Build history of the part. All positions in model axes, mm. A direction names the side the tool comes from. Round coordinates to 2 decimals unless told otherwise and drop trailing zeros. Loops run counter-clockwise (first coordinate to the right, second up) from the corner with the lowest first, then second, coordinate; pieces in that order, holes last. Notation, with made-up numbers: (21.25, 42.25) -> (40.25, 42.25) arc R14 cw to (40.25, 59.25) -> close; hole circle Ø9 at (-6.75, 19). An arc over 180 degrees is marked (long way). Put each result on its own line as item: value. Start each with the question number.
Item 1: Cut at A-A, the plane y = 0. List the corners of the cut face in (x, z), plus the area to 3 significant figures.
Item 2: Cut at C-C, the plane z = 0.75. Count the separate pieces of the cut face and the enclosed holes in it, plus the area to 3 significant figures.
Item 3: Tool access for faces 4 (the cylindrical face through (-2.664, -13.159, 1.479)), 5 (the cylindrical face through (-11.995, -5.952, 1.479)), 6 (the flat face through (8, 2, 3)), 7 (the flat face through (8.631, -0.183, 1.479)): list every direction of +Z, -Z, +X, -X, +Y, -Y with a clear straight run to the whole face (end or side of a thin tool).
Item 4: Cut at B-B, the plane x = 11. List the corners of the cut face in (y, z).
Item 5: Pull direction Y, two halves, no side cores. Call faces 1 (the cylindrical face through (-10.046, -8.853, 1.479)), 2 (the flat face through (37.972, -12.897, 1.479)), 3 (the flat face through (27.025, -3.925, 1.479)): +Y half, -Y half, draft (parallel to the pull), parting line (faces both ways), or undercut.
Item 6: Drill centre lines: probe 1 along Y at (x, z) = (20, 0.35); probe 2 along X at (y, z) = (0, 1.25); probe 3 along X at (y, z) = (2.75, 2.7). Where is each one in solid material? Low to high. Write a range as [from, to].
Item 7: Flat gauge pins, fed straight in: pin 1 Ø1 at (x, z) = (20, 2) entering from +Y; pin 2 Ø0.9 at (x, z) = (21, 1.5) entering from -Y; pin 3 Ø1 at (y, z) = (-6.5, 1.5) entering from -X; pin 4 Ø2.5 at (x, y) = (41.23, -11.45) entering from -Z. Where does each tip first touch, or does it go through?
```python
from build123d import *

# Parameters (mm, degrees)
SKETCH2_R           = 1.5
BOSS_EXTRUDE2_DEPTH = 3
CUT_EXTRUDE2_DEPTH  = 3


with BuildPart() as part:
    # Sketch2 → Boss-Extrude2 (new body)
    with BuildSketch(Plane.XY):
        with BuildLine():
            Line((33.856406461, -4.911436862), (20, -2.911436862))
            Line((20, -2.911436862), (8.072676136, 9))
            ThreePointArc((8.072676136, 9), (-5.877422545, 10.565226179), (-11.903927815, -2.112960617))
            ThreePointArc((-11.903927815, -2.112960617), (-13.14288127, -2.654199937), (-14.208555951, -3.486235477))
            ThreePointArc((-14.208555951, -3.486235477), (-14.131494839, -3.78652263), (-14.048088143, -4.085109489))
            ThreePointArc((-14.048088143, -4.085109489), (-12.709169027, -4.272836063), (-11.365584201, -4.122086336))
            ThreePointArc((-11.365584201, -4.122086336), (-11.169703548, -4.626642697), (-10.951436862, -5.12192646))
            ThreePointArc((-10.951436862, -5.12192646), (-12.008090957, -5.965388247), (-12.82210701, -7.044889767))
            ThreePointArc((-12.82210701, -7.044889767), (-12.669951657, -7.315), (-12.51210701, -7.581825517))
            ThreePointArc((-12.51210701, -7.581825517), (-11.170223244, -7.416617696), (-9.911436862, -6.9232593))
            ThreePointArc((-9.911436862, -6.9232593), (-9.591641884, -7.359925677), (-9.252623584, -7.781841479))
            ThreePointArc((-9.252623584, -7.781841479), (-10.05496909, -8.870045207), (-10.561852666, -10.123446462))
            ThreePointArc((-10.561852666, -10.123446462), (-10.344972209, -10.344972209), (-10.123446462, -10.561852666))
            ThreePointArc((-10.123446462, -10.561852666), (-8.870045207, -10.05496909), (-7.781841479, -9.252623584))
            ThreePointArc((-7.781841479, -9.252623584), (-7.359925677, -9.591641884), (-6.9232593, -9.911436862))
            ThreePointArc((-6.9232593, -9.911436862), (-7.416617696, -11.170223244), (-7.581825517, -12.51210701))
            ThreePointArc((-7.581825517, -12.51210701), (-7.315, -12.669951657), (-7.044889767, -12.82210701))
            ThreePointArc((-7.044889767, -12.82210701), (-5.965388247, -12.008090957), (-5.12192646, -10.951436862))
            ThreePointArc((-5.12192646, -10.951436862), (-4.626642697, -11.169703548), (-4.122086336, -11.365584201))
            ThreePointArc((-4.122086336, -11.365584201), (-4.272836063, -12.709169027), (-4.085109489, -14.048088143))
            ThreePointArc((-4.085109489, -14.048088143), (-3.78652263, -14.131494839), (-3.486235477, -14.208555951))
            ThreePointArc((-3.486235477, -14.208555951), (-2.654199937, -13.14288127), (-2.112960617, -11.903927815))
            ThreePointArc((-2.112960617, -11.903927815), (-1.578061664, -11.986568374), (-1.04, -12.04518576))
            ThreePointArc((-1.04, -12.04518576), (-0.837867713, -13.382005944), (-0.31, -14.626715284))
            ThreePointArc((-0.31, -14.626715284), (0, -14.63), (0.31, -14.626715284))
            ThreePointArc((0.31, -14.626715284), (0.837867713, -13.382005944), (1.04, -12.04518576))
            ThreePointArc((1.04, -12.04518576), (1.578061664, -11.986568374), (2.112960617, -11.903927815))
            ThreePointArc((2.112960617, -11.903927815), (2.654199937, -13.14288127), (3.486235477, -14.208555951))
            ThreePointArc((3.486235477, -14.208555951), (3.78652263, -14.131494839), (4.085109489, -14.048088143))
            ThreePointArc((4.085109489, -14.048088143), (4.272836063, -12.709169027), (4.122086336, -11.365584201))
            ThreePointArc((4.122086336, -11.365584201), (4.626642697, -11.169703548), (5.12192646, -10.951436862))
            ThreePointArc((5.12192646, -10.951436862), (5.965388247, -12.008090957), (7.044889767, -12.82210701))
            ThreePointArc((7.044889767, -12.82210701), (7.315, -12.669951657), (7.581825517, -12.51210701))
            ThreePointArc((7.581825517, -12.51210701), (7.416617696, -11.170223244), (6.9232593, -9.911436862))
            ThreePointArc((6.9232593, -9.911436862), (7.51180399, -9.473167412), (8.072676136, -9))
            Line((8.072676136, -9), (16, -11.911436862))
            Line((16, -11.911436862), (36, -11.911436862))
            Line((36, -11.911436862), (40, -13.911436862))
            ThreePointArc((40, -13.911436862), (43.70240259, -12.65581862), (42.40824957, -8.966708962))
            Line((42.40824957, -8.966708962), (33.856406461, -4.911436862))
        make_face()
        with Locations((41.229904242, -11.451628378)):
            Circle(SKETCH2_R, mode=Mode.SUBTRACT)
    extrude(amount=BOSS_EXTRUDE2_DEPTH)

    # Sketch4 → Cut-Extrude2 (cut)
    with BuildSketch(Plane(origin=(0, 0, 0), x_dir=(-1, 0, 0), z_dir=(0, 0, -1))):
        with BuildLine():
            Line((-1.721055129, 3.358246048), (-15.737581702, -3.825031953))
            ThreePointArc((-15.737581702, -3.825031953), (-16.698373457, -6.319012023), (-14.327181541, -7.55210013))
            Line((-14.327181541, -7.55210013), (0.933399378, -3.656311376))
            ThreePointArc((0.933399378, -3.656311376), (3.529320665, 1.335568388), (-1.721055129, 3.358246048))
        make_face()
    extrude(amount=-CUT_EXTRUDE2_DEPTH, mode=Mode.SUBTRACT)


solid = part.part
```
Reply:
1. outline: (-12.09, 0) -> (-3.77, 0) -> (-3.77, 3) -> (-12.09, 3) -> close; (8.27, 0) -> (17.08, 0) -> (17.08, 3) -> (8.27, 3) -> close
1. area: 51.4 mm^2
2. separate pieces: 1
2. enclosed holes: 2
2. area: 649 mm^2
3. face 4: +Z, -Z, -Y
3. face 5: +Z, -Z, -X
3. face 6: +Z, +X, -X, +Y, -Y
3. face 7: +Z, -Z
4. outline: (-10.08, 0) -> (-6.7, 0) -> (-6.7, 3) -> (-10.08, 3) -> close; (-1.4, 0) -> (6.08, 0) -> (6.08, 3) -> (-1.4, 3) -> close
5. face 1: undercut
5. face 2: -Y half
5. face 3: +Y half
6. probe 1: y = [-11.91, -2.91]
6. probe 2: x = [-12.09, -3.77], [8.27, 17.08]
6. probe 3: x = [-11.77, -2.58], [2.91, 14.33]
7. pin 1: stops at y = -2.41
7. pin 2: stops at y = -11.91
7. pin 3: stops at x = -12.8
7. pin 4: passes through
